Read the model definition and answer for the solid it produces. Units are mm, in the model's axes. Coordinates: 2 decimals unless noted, no trailing zeros. Order: outer loops, then holes, each group sorted by start corner. A loop starts at its lowest first (then second) coordinate and runs counter-clockwise, first axis right, second up. Notation, with made-up numbers: M 38.5,-27.5 L 89.5,-27.5 A11 cw 89.5,-22.5 Z; hole C -24.75,-24 d7. An arc over 180 degrees is marked long. Put each result on its own line as item: value.
from build123d import *

# Parameters (mm, degrees)
EXTRUDE_THIN1_DEPTH = 254
FILLET1_R           = 1.016


with BuildPart() as part:
    # Sketch1 → Extrude-Thin1 (new body)
    with BuildSketch(Plane.XY):
        with BuildLine():
            Line((0, 0), (-5.55625, 0))
            Line((-5.55625, 0), (-5.55625, 4.7625))
            Line((-5.55625, 4.7625), (-7.9375, 4.7625))
            ThreePointArc((-7.9375, 4.7625), (-9.323959524, 14.156943651), (-17.4625, 19.05))
            Line((-17.4625, 19.05), (-17.4625, 25.4))
            Line((-17.4625, 25.4), (0, 25.4))
            Line((0, 25.4), (0, 24.384))
            Line((0, 24.384), (-16.4465, 24.384))
            Line((-16.4465, 24.384), (-16.4465, 19.933974896))
            ThreePointArc((-16.4465, 19.933974896), (-8.598518146, 14.89701763), (-6.645470806, 5.7785))
            Line((-6.645470806, 5.7785), (-4.54025, 5.7785))
            Line((-4.54025, 5.7785), (-4.54025, 1.016))
            Line((-4.54025, 1.016), (0, 1.016))
            Line((0, 1.016), (0, 0))
        make_face()
    extrude(amount=-EXTRUDE_THIN1_DEPTH)

    # Fillet1
    fillet1_edges = [part.edges().sort_by_distance(p)[0] for p in [
        (-4.54025, 5.7785, -127),
        (-5.55625, 0, -127),
        (-7.9375, 4.7625, -127),
        (-17.4625, 19.05, -127),
        (-17.4625, 25.4, -127),
    ]]
    fillet(fillet1_edges, radius=FILLET1_R)


solid = part.part
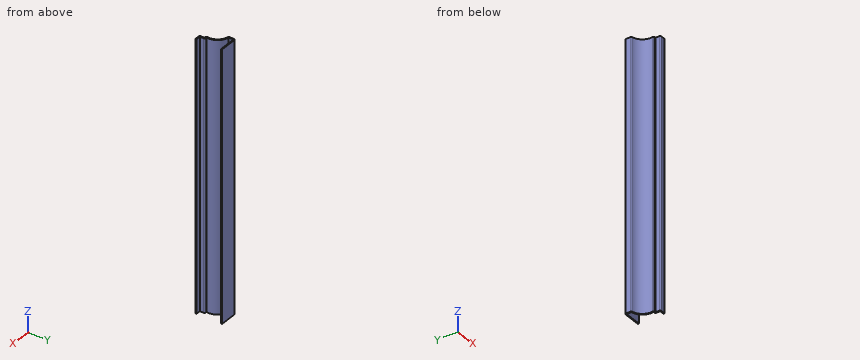
Q1. Find section C-C on y = 15.25. Write down the section's boundary in (x, z).
Answers below:
outline: M -10.15,-254 L -8.85,-254 L -8.85,0 L -10.15,0 Z
Q2. Find section B-B on z = -218. Write down the section's boundary in (x, y) (1 decimal), plus the area to 3 significant figures.
Answers below:
outline: M -17.5,19.9 A1 ccw -16.6,18.9 A11.1 cw -7.6,6 A1 ccw -6.6,4.8 L -5.6,4.8 L -5.6,1 A1 ccw -4.5,0 L 0,0 L 0,1 L -4.5,1 L -4.5,4.8 A1 ccw -5.6,5.8 L -6.6,5.8 A12.1 ccw -16.4,19.9 L -16.4,24.4 L 0,24.4 L 0,25.4 L -16.4,25.4 A1 ccw -17.5,24.4 Z
area: 53.4 mm^2
Q3. Consider line 1 along Y through (x, z) = (-5.75, -113.5); line 2 along Y through (x, z) = (-1.5, -64.5); line 3 along X through (y, z) = (23.25, -30.5). Determine where each line is inside the solid, lowest interval first.
Answers below:
line 1: y = 4.76 to 5.78, 24.38 to 25.4
line 2: y = 0 to 1.02, 24.38 to 25.4
line 3: x = -17.46 to -16.45
Q4. Given pin 1 (1.5 mm diameter, centred on x = -10, z = -200.5, fed in from -Y); pin 2 (2 mm diameter, centred on y = 21.5, z = -97.5, fed in from +X); pin 3 (10 mm diameter, centred on y = 8, z = -96, fed in from +X); pin 4 (6 mm diameter, centred on x = -6.5, y = 17.5, fed in from -Z), each flat-ended and moving along its own axis, determine where each tip first touches the part or whether it passes through.
Answers below:
pin 1: stops at y = 14.04
pin 2: stops at x = -16.45
pin 3: stops at x = -4.54
pin 4: passes through
Q5. Find section A-A on x = -13.75. Write down the section's boundary in (y, z).
Answers below:
outline: M 18.01,-254 L 19.12,-254 L 19.12,0 L 18.01,0 Z; M 24.38,-254 L 25.4,-254 L 25.4,0 L 24.38,0 Z
